from build123d import *

# Parameters (mm, degrees)
BOSS_EXTRUDE5_DEPTH = 10
BOSS_EXTRUDE6_DEPTH = 14.5
BOSS_EXTRUDE7_REACH = 63.425
SKETCH28_W          = 11
SKETCH28_H          = 29
SKETCH37_W          = 23.2
SKETCH37_H          = 14.666666667
CUT_EXTRUDE10_DEPTH = 6
SKETCH38_W          = 23.2
SKETCH38_H          = 5
CUT_EXTRUDE11_DEPTH = 6
SKETCH39_R          = 1.05
CUT_EXTRUDE12_DEPTH = 81.736980805
SKETCH40_R          = 2
CUT_EXTRUDE13_DEPTH = 1.4
SKETCH41_R          = 2
CUT_EXTRUDE14_DEPTH = 1.4
SKETCH42_W          = 17
SKETCH42_H          = 40
CUT_EXTRUDE15_DEPTH = 77.175521458
FILLET2_R           = 2
CUT_EXTRUDE16_DEPTH = 80.232001549
BOSS_EXTRUDE8_DEPTH = 10
FILLET3_R           = 10


with BuildPart() as part:
    # Sketch25 → Boss-Extrude5 (new, symmetric)
    with BuildSketch(Plane.XY):
        with BuildLine():
            Line((0, 15.875), (6.35, 15.875))
            ThreePointArc((6.35, 15.875), (9.840958299, 0), (6.35, -15.875))
            Line((6.35, -15.875), (0, -15.875))
            ThreePointArc((0, -15.875), (4.187196601, 0), (0, 15.875))
        make_face()
    extrude(amount=BOSS_EXTRUDE5_DEPTH, both=True)


with BuildPart() as body_2:
    # Sketch27 → Boss-Extrude6 (new, symmetric)
    with BuildSketch(Plane.XY):
        Polygon((0, -30.541666667), (11, -30.541666667), (11, -74.541666667), (0, -74.541666667), (0, -69.541666667), (6, -69.541666667), (6, -35.541666667), (0, -35.541666667), align=None)
    extrude(amount=BOSS_EXTRUDE6_DEPTH, both=True)

    # Sketch28 → Boss-Extrude7 (add, up to next)
    with BuildSketch(Plane.XZ.offset(15.875), mode=Mode.PRIVATE) as boss_extrude7_sk1:
        with Locations((5.5, 0)):
            Rectangle(SKETCH28_W, SKETCH28_H)
    boss_extrude7_tool1 = extrude(boss_extrude7_sk1.sketch, amount=BOSS_EXTRUDE7_REACH, mode=Mode.PRIVATE) - body_2.part

    add(part.part)  # Boss-Extrude7 merges part
    add(boss_extrude7_tool1.solids().sort_by_distance((5.5, -15.875, 0))[0])

    # Sketch37 → Cut-Extrude10 (cut)
    with BuildSketch(Plane.ZY):
        with Locations((0, -28.208333334)):
            Rectangle(SKETCH37_W, SKETCH37_H)
    extrude(amount=-CUT_EXTRUDE10_DEPTH, mode=Mode.SUBTRACT)

    # Sketch38 → Cut-Extrude11 (cut)
    with BuildSketch(Plane.ZY):
        with Locations((0, -72.041666667)):
            Rectangle(SKETCH38_W, SKETCH38_H)
    extrude(amount=-CUT_EXTRUDE11_DEPTH, mode=Mode.SUBTRACT)

    # Sketch39 → Cut-Extrude12 (cut, through all)
    with BuildSketch(Plane(origin=(0, 0, -14.5), x_dir=(-1, 0, 0), z_dir=(0, 0, -1))):
        with Locations((-2.5, -33.041666667)):
            Circle(SKETCH39_R)
        with Locations((-2.5, -72.041666667)):
            Circle(SKETCH39_R)
    extrude(amount=-CUT_EXTRUDE12_DEPTH, mode=Mode.SUBTRACT)

    # Sketch40 → Cut-Extrude13 (cut)
    with BuildSketch(Plane(origin=(0, 0, -14.5), x_dir=(-1, 0, 0), z_dir=(0, 0, -1))):
        with Locations((-2.5, -33.041666667)):
            Circle(SKETCH40_R)
        with Locations((-2.5, -72.041666667)):
            Circle(SKETCH40_R)
    extrude(amount=-CUT_EXTRUDE13_DEPTH, mode=Mode.SUBTRACT)

    # Sketch41 → Cut-Extrude14 (cut)
    with BuildSketch(Plane.XY.offset(14.5)):
        with Locations(Location((2.5, -33.041666667, 0), (0, 0, 180))):
            Circle(SKETCH41_R)
        with Locations(Location((2.5, -72.041666667, 0), (0, 0, 180))):
            Circle(SKETCH41_R)
    extrude(amount=-CUT_EXTRUDE14_DEPTH, mode=Mode.SUBTRACT)

    # Sketch42 → Cut-Extrude15 (cut, through all)
    with BuildSketch(Plane.ZY.offset(-6)):
        with Locations((0, -49.541666667)):
            Rectangle(SKETCH42_W, SKETCH42_H)
    extrude(amount=-CUT_EXTRUDE15_DEPTH, mode=Mode.SUBTRACT)

    # Fillet2
    fillet2_edges = [body_2.edges().sort_by_distance(p)[0] for p in [
        (8.5, -69.541666667, -8.5),
        (8.5, -29.541666667, -8.5),
        (8.5, -29.541666667, 8.5),
        (8.5, -69.541666667, 8.5),
        (0, -35.541666667, 13.05),
        (0, -69.541666667, 13.05),
        (0, -74.541666667, 13.05),
        (11, -74.541666667, 0),
        (0, -35.541666667, -13.05),
        (0, -74.541666667, -13.05),
        (0, -69.541666667, -13.05),
    ]]
    fillet(fillet2_edges, radius=FILLET2_R)

    # Sketch44 → Cut-Extrude16 (cut, through all)
    with BuildSketch(Plane.XY.offset(10)):
        with BuildLine():
            Line((6.35, -15.875), (0, -15.875))
            ThreePointArc((0, -15.875), (4.187196601, 0), (0, 15.875))
            Line((0, 15.875), (6.35, 15.875))
            ThreePointArc((6.35, 15.875), (9.840958299, 0), (6.35, -15.875))
        make_face()
    extrude(amount=-CUT_EXTRUDE16_DEPTH, mode=Mode.SUBTRACT)

    # Sketch43 → Boss-Extrude8 (add, symmetric)
    with BuildSketch(Plane.XY):
        with BuildLine():
            Line((-3.25, 15.875), (3.1, 15.875))
            ThreePointArc((3.1, 15.875), (6.232422098, 0), (3.1, -15.875))
            Line((3.1, -15.875), (-3.25, -15.875))
            ThreePointArc((-3.25, -15.875), (0.439252949, 0), (-3.25, 15.875))
        make_face()
    extrude(amount=BOSS_EXTRUDE8_DEPTH, both=True)

    # Fillet3
    # the kernel refuses this fillet: 10 mm, written as the material it takes off along each edge
    with BuildSketch(Plane(origin=(11, -15.875, 39.5), x_dir=(-1, 0, 0), z_dir=(0, 0, -1))) as fillet3_piece_1_section:
        with BuildLine():
            CenterArc((FILLET3_R, -FILLET3_R), FILLET3_R, 90, 90)
            Line((0, -FILLET3_R), (0, 0))
            Line((0, 0), (FILLET3_R, 0))
        make_face()
    fillet3_piece_1 = extrude(amount=79, mode=Mode.PRIVATE)
    fillet3_piece_1 = split(fillet3_piece_1, bisect_by=Plane(origin=(2.190951885, -15.815672455, 10), z_dir=(0, 0, 1)), keep=Keep.TOP, mode=Mode.PRIVATE)
    fillet3_piece_1 = fillet3_piece_1 & Plane(origin=(-35.560747051, 0, 24.75), x_dir=(0.925049424055658, 0.3798467625955178, 0), z_dir=(0, 0, 1)) * Cylinder(41.793169149, 198, mode=Mode.PRIVATE)
    add(fillet3_piece_1, mode=Mode.SUBTRACT)
    with BuildSketch(Plane(origin=(11, -15.875, 39.5), x_dir=(-1, 0, 0), z_dir=(0, 0, -1))) as fillet3_piece_2_section:
        with BuildLine():
            CenterArc((FILLET3_R, -FILLET3_R), FILLET3_R, 90, 90)
            Line((0, -FILLET3_R), (0, 0))
            Line((0, 0), (FILLET3_R, 0))
        make_face()
    fillet3_piece_2 = extrude(amount=79, mode=Mode.PRIVATE)
    fillet3_piece_2 = split(fillet3_piece_2, bisect_by=Plane(origin=(8.886802667, -18.192463431, 10), z_dir=(0, 0, 1)), keep=Keep.TOP, mode=Mode.PRIVATE)
    fillet3_piece_2 = fillet3_piece_2 - Plane(origin=(-35.560747051, 0, 24.75), x_dir=(0.925049424055658, 0.3798467625955178, 0), z_dir=(0, 0, 1)) * Cylinder(41.793169149, 198, mode=Mode.PRIVATE)
    add(fillet3_piece_2, mode=Mode.SUBTRACT)
    with BuildSketch(Plane(origin=(11, -15.875, 39.5), x_dir=(-1, 0, 0), z_dir=(0, 0, -1))) as fillet3_piece_3_section:
        with BuildLine():
            CenterArc((FILLET3_R, -FILLET3_R), FILLET3_R, 90, 90)
            Line((0, -FILLET3_R), (0, 0))
            Line((0, 0), (FILLET3_R, 0))
        make_face()
    fillet3_piece_3 = extrude(amount=79, mode=Mode.PRIVATE)
    fillet3_piece_3 = split(fillet3_piece_3, bisect_by=Plane(origin=(8.886802667, -18.192463431, 10), z_dir=(0, 0, -1)), keep=Keep.TOP, mode=Mode.PRIVATE)
    fillet3_piece_3 = fillet3_piece_3 - Plane(origin=(-35.560747051, 0, 0), x_dir=(0.925049424055658, 0.3798467625955178, 0), z_dir=(0, 0, 1)) * Cylinder(41.793169149, 198, mode=Mode.PRIVATE)
    fillet3_piece_3 = split(fillet3_piece_3, bisect_by=Plane(origin=(8.886802667, -18.192463431, -10), z_dir=(0, 0, 1)), keep=Keep.TOP, mode=Mode.PRIVATE)
    add(fillet3_piece_3, mode=Mode.SUBTRACT)
    with BuildSketch(Plane(origin=(11, -15.875, 39.5), x_dir=(-1, 0, 0), z_dir=(0, 0, -1))) as fillet3_piece_4_section:
        with BuildLine():
            CenterArc((FILLET3_R, -FILLET3_R), FILLET3_R, 90, 90)
            Line((0, -FILLET3_R), (0, 0))
            Line((0, 0), (FILLET3_R, 0))
        make_face()
    fillet3_piece_4 = extrude(amount=79, mode=Mode.PRIVATE)
    fillet3_piece_4 = fillet3_piece_4 & Plane(origin=(-35.560747051, 0, -24.75), x_dir=(0.925049424055658, 0.3798467625955178, 0), z_dir=(0, 0, 1)) * Cylinder(41.793169149, 198, mode=Mode.PRIVATE)
    fillet3_piece_4 = split(fillet3_piece_4, bisect_by=Plane(origin=(2.190951885, -15.815672455, -10), z_dir=(0, 0, -1)), keep=Keep.TOP, mode=Mode.PRIVATE)
    add(fillet3_piece_4, mode=Mode.SUBTRACT)
    with BuildSketch(Plane(origin=(11, -15.875, 39.5), x_dir=(-1, 0, 0), z_dir=(0, 0, -1))) as fillet3_piece_5_section:
        with BuildLine():
            CenterArc((FILLET3_R, -FILLET3_R), FILLET3_R, 90, 90)
            Line((0, -FILLET3_R), (0, 0))
            Line((0, 0), (FILLET3_R, 0))
        make_face()
    fillet3_piece_5 = extrude(amount=79, mode=Mode.PRIVATE)
    fillet3_piece_5 = fillet3_piece_5 - Plane(origin=(-35.560747051, 0, -24.75), x_dir=(0.925049424055658, 0.3798467625955178, 0), z_dir=(0, 0, 1)) * Cylinder(41.793169149, 198, mode=Mode.PRIVATE)
    fillet3_piece_5 = split(fillet3_piece_5, bisect_by=Plane(origin=(8.886802667, -18.192463431, -10), z_dir=(0, 0, -1)), keep=Keep.TOP, mode=Mode.PRIVATE)
    add(fillet3_piece_5, mode=Mode.SUBTRACT)


solid = body_2.part
Work out the finished part from the listing and answer in its coordinate system (mm). A direction names the side the tool comes from. Round coordinates to 2 decimals unless told otherwise and drop trailing zeros. Write each loop counter-clockwise with the first axis right and the second up, starting at its lowest first coordinate (ties: lowest second). Pieces come first, ordered by that corner, then holes. Notation, with made-up numbers: (-8.75, 28.25) - (5.25, 28.25) arc R9 ccw to (5.25, 39.25) - close; hole circle Ø8 at (13, 25). An arc over 180 degrees is marked (long way). Answer in a Markdown table with one row per item. Add a question column.
1. A cutting plane is placed at B-B, the plane x = 10. Determine the outline of the cut face in (y, z).
2. The mould has two halves that part along X. Classify faces 1 (the cylindrical face through (2.64, -32, -12.36)), 2 (the cylindrical face through (0.57, -70.143, -13.07)), 3 (the flat face through (7, -45, 14.5)): +X half, -X half, draft (parallel to the pull), parting line (faces both ways), or undercut.
3. Given pin 1 (4 mm diameter, centred on x = 2.5, y = -71.5, fed in from +Z); pin 2 (4 mm diameter, centred on y = -1.5, z = 8.5, fed in from +X); pin 3 (1.1 mm diameter, centred on y = -72, z = 12.5, fed in from -X); pin 4 (1.1 mm diameter, centred on x = 0.5, z = 13, fed in from +Y) (3 decimals), each flat-ended and moving along its own axis, determine where each tip first touches the part or whether it passes through.
4. For faces 4 (the cylindrical face through (1.425, -73.728, 13.81)), 5 (the flat face through (4, -72, 11.6)), 6 (the cylindrical face through (8.535, -30.143, 7.93)), determine the directions among +Z, -Z, +X, -X, +Y, -Y from which every point of the face is accessible in a straight line to the end or side of a thin tool.
5. Find the intervals of material crossed by line 1 along Y through (x, z) = (2.5, -14.15); line 2 along Y through (x, z) = (2.5, 12.4); line 3 along Y through (x, z) = (2.75, 9.75) (3 decimals), in increasing order. Write a range as from..to.
6. A cutting plane is placed at A-A, the plane z = -3.75. Determine the outline of the cut face in (x, y) (3 decimals), and give its area (3 significant figures).
7. A cutting plane is placed at C-C, the plane y = -13.5. Determine the outline of the cut face in (x, z), and give its area (3 significant figures).
Worked out:
| question | item | result |
|---|---|---|
| 1 | outline | (-74.27, -14.5) - (-21.52, -14.5) - (-21.52, 14.5) - (-74.27, 14.5) - close; hole (-69.54, -6.5) arc R2 ccw to (-67.54, -8.5) - (-31.54, -8.5) arc R2 ccw to (-29.54, -6.5) - (-29.54, 6.5) arc R2 ccw to (-31.54, 8.5) - (-67.54, 8.5) arc R2 ccw to (-69.54, 6.5) - close |
| 2 | face 1 | undercut |
| 2 | face 2 | -X half |
| 2 | face 3 | draft |
| 3 | pin 1 | z = 14.5 |
| 3 | pin 2 | x = 6.23 |
| 3 | pin 3 | x = 0 |
| 3 | pin 4 | y = -15.875 |
| 4 | face 4 | +Z |
| 4 | face 5 | -X, -Y |
| 4 | face 6 | +X, -X |
| 5 | line 1 | -74.54..-74.04, -70.04..-69.54, -35.54..-35.04, -31.04..-15.99 |
| 5 | line 2 | -74.54..-73.09, -70.99..-69.54, -35.54..-34.09, -31.99..-15.99 |
| 5 | line 3 | -20.875..15.875 |
| 6 | outline | (-3.25, -15.875) - (0, -15.875) - (0, -20.875) - (6, -20.875) - (6, -29.542) - (11, -29.542) - (11, -25.875) arc R10 ccw to (3.015, -16.08) arc R41.793 ccw to (3.1, 15.875) - (-3.25, 15.875) arc R36 cw to start; (6, -74.542) - (9, -74.542) arc R2 ccw to (11, -72.542) - (11, -69.542) - (6, -69.542) - close |
| 6 | area | 291 mm^2 |
| 7 | outline | (-2.19, -10) - (3.99, -10) - (3.99, 10) - (-2.19, 10) - close |
| 7 | area | 124 mm^2 |
